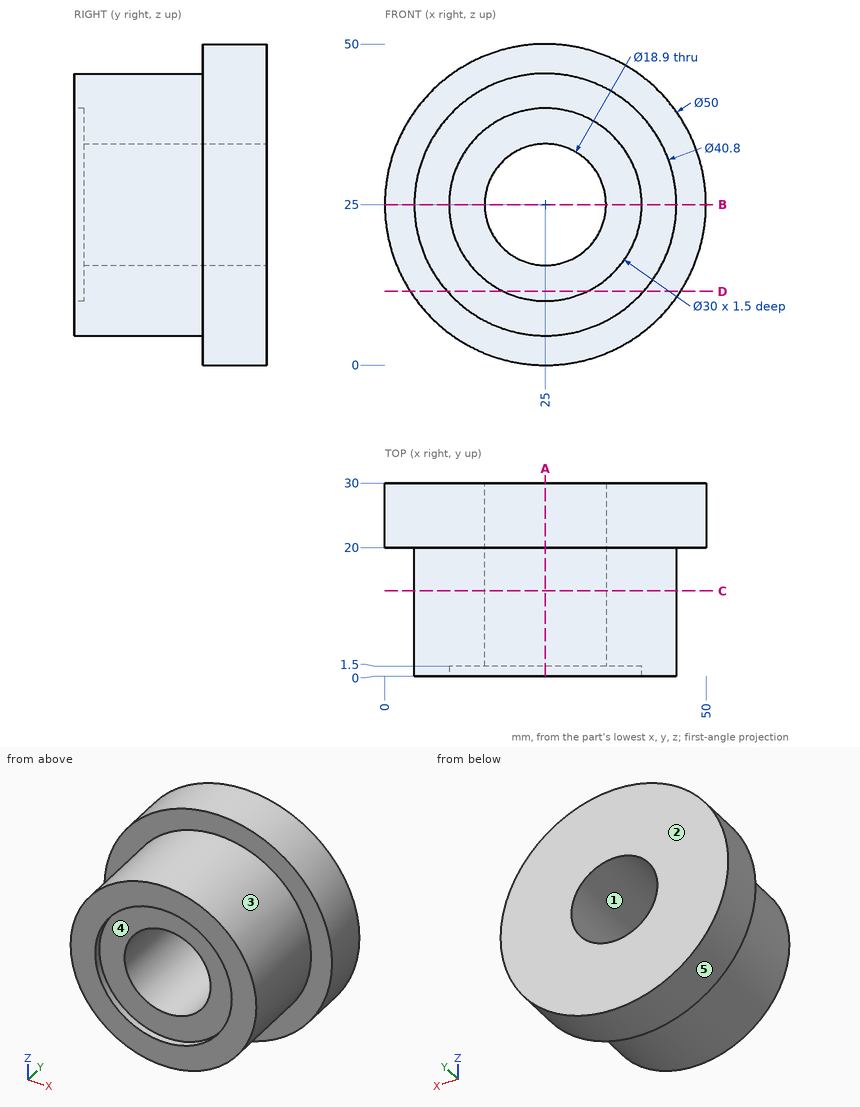
The drawing under review shows one solid part. Ordinate dimensions are in mm from its lowest x, y, z. A direction names the side the tool comes from. Coordinates: 2 decimals unless noted, no trailing zeros. Loops run counter-clockwise (first coordinate to the right, second up) from the corner with the lowest first, then second, coordinate; pieces in that order, holes last. Notation, with made-up numbers: (23.25, 44.25) - (67.25, 44.25) arc R27 cw to (67.25, 79.25) - close; hole circle Ø2 at (33, 13). An arc over 180 degrees is marked (long way). Return JSON: item names as keys, results as strings.
Item 1: Insertion check: pin 1 (4 mm diameter, centred on y = 24.5, z = 20, fed in from -X); pin 2 (24 mm diameter, centred on x = 25, z = 25, fed in from -Y); pin 3 (10 mm diameter, centred on x = 36, y = 23.5, fed in from -Z); pin 4 (17 mm diameter, centred on x = 25, z = 25, fed in from -Y) (1 decimal). Each pin has a flat end and moves straight along its axis. Give the tip position at first contact, or say it passes through.
Determined:
{"pin 1": "stops at x = 0.18", "pin 2": "stops at y = 1.5", "pin 3": "stops at z = 0.73", "pin 4": "passes through"}
Item 2: For the marked faces 4 and 5, list the 3-axis set-ups (+Z, -Z, +X, -X, +Y, -Y) from which the entire face can be reached by the end or side of a thin tool; tool diameter is ignored.
Determined:
{"face 4": "-Y", "face 5": "+Y, -Y"}
Item 3: Take a section at A-A (x = 25). Give the boundary of the cut face in (y, z), then the cut area to 3 significant figures.
Determined:
{"outline": "(0, 4.6) - (20, 4.6) - (20, 0) - (30, 0) - (30, 15.55) - (1.5, 15.55) - (1.5, 10) - (0, 10) - close; (0, 40) - (1.5, 40) - (1.5, 34.45) - (30, 34.45) - (30, 50) - (20, 50) - (20, 45.4) - (0, 45.4) - close", "area": "732 mm2"}
Item 4: Take a section at D-D (z = 11.5). Give the boundary of the cut face in (x, y).
Determined:
{"outline": "(3.96, 20) - (9.71, 20) - (9.71, 0) - (18.46, 0) - (18.46, 1.5) - (31.54, 1.5) - (31.54, 0) - (40.29, 0) - (40.29, 20) - (46.04, 20) - (46.04, 30) - (3.96, 30) - close"}
Item 5: Take a section at B-B (z = 25). Give the boundary of the cut face in (x, y), then the cut area to 3 significant figures.
Determined:
{"outline": "(0, 20) - (4.6, 20) - (4.6, 0) - (10, 0) - (10, 1.5) - (15.55, 1.5) - (15.55, 30) - (0, 30) - close; (34.45, 1.5) - (40, 1.5) - (40, 0) - (45.4, 0) - (45.4, 20) - (50, 20) - (50, 30) - (34.45, 30) - close", "area": "732 mm2"}
Item 6: For line 1 (Z direction, x = 25, y = 0.6); line 2 (Z direction, x = 25, y = 15.25); line 3 (Y direction, x = 47, z = 24), list the stretches that pass through material, from the lowest coordinate up.
Determined:
{"line 1": "z = 4.6 to 10, 40 to 45.4", "line 2": "z = 4.6 to 15.55, 34.45 to 45.4", "line 3": "y = 20 to 30"}
Item 7: Mouldability with a two-part tool opening along Z and no side actions: class the marked faces 1, 2 and 3 as pulls with the +Z half, pulls with the -Z half, needs draft (parallel to the pull), parting line crosses it, or undercut.
Determined:
{"face 1": "undercut", "face 2": "needs draft", "face 3": "parting line crosses it"}
Item 8: Take a section at C-C (y = 13.25). Give the boundary of the cut face in (x, z).
Determined:
{"outline": "circle Ø40.8 at (25, 25); hole circle Ø18.9 at (25, 25)"}
